```python
from build123d import *

# Parameters (mm, degrees)
SKETCH1_W                = 75
SKETCH1_H                = 40
SKETCH1_R                = 5
SKETCH1_R_2              = 1.7
SKETCH1_R_3              = 1.197563381
SKETCH1_W_2              = 5
SKETCH1_H_2              = 20
BOSS_EXTRUDE1_DEPTH      = 3
CUT_EXTRUDE1_DEPTH       = 43.605750786
CUT_EXTRUDE1_DEPTH_BACK  = 43.605750786
SKETCH2_W                = 67
SKETCH2_H                = 28
BOSS_EXTRUDE3_DEPTH      = 75
BOSS_EXTRUDE3_DEPTH_BACK = 3
SKETCH6_W                = 67
SKETCH6_H                = 11
CUT_EXTRUDE4_DEPTH       = 91.863909227
SKETCH7_W                = 70
SKETCH7_H                = 37
BOSS_EXTRUDE4_DEPTH      = 6
SKETCH8_W                = 6
SKETCH8_H                = 62
CUT_EXTRUDE6_DEPTH       = 29
SKETCH9_R                = 1.25
SKETCH9_R_2              = 10.5
CUT_EXTRUDE8_DEPTH       = 122.975407357
SKETCH11_W               = 6
SKETCH11_H               = 4
CUT_EXTRUDE9_DEPTH       = 114.473565204
SKETCH12_W               = 35
SKETCH12_H               = 4
BOSS_EXTRUDE5_DEPTH      = 70
SKETCH13_R               = 5
SKETCH13_R_2             = 1.7
CUT_EXTRUDE11_DEPTH      = 10


with BuildPart() as part:
    # Sketch1 → Boss-Extrude1 (new body)
    with BuildSketch(Plane(origin=(0, 0, 0), x_dir=(1, 0, 0), z_dir=(0, 1, 0))):
        Rectangle(SKETCH1_W, SKETCH1_H)
        with Locations(Location((-21, 0, 0), (0, 0, 270))):
            Circle(SKETCH1_R, mode=Mode.SUBTRACT)
        with Locations(Location((-30, 8.25, 0), (0, 0, 270))):
            Circle(SKETCH1_R_2, mode=Mode.SUBTRACT)
        with Locations(Location((-12, 8.25, 0), (0, 0, 270))):
            Circle(SKETCH1_R_2, mode=Mode.SUBTRACT)
        with Locations(Location((-12, -8.25, 0), (0, 0, 270))):
            Circle(SKETCH1_R_2, mode=Mode.SUBTRACT)
        with Locations(Location((-30, -8.25, 0), (0, 0, 270))):
            Circle(SKETCH1_R_2, mode=Mode.SUBTRACT)
        with Locations(Location((12, 8.25, 0), (0, 0, 90))):
            Circle(SKETCH1_R_2, mode=Mode.SUBTRACT)
        with Locations(Location((12, -8.25, 0), (0, 0, 90))):
            Circle(SKETCH1_R_2, mode=Mode.SUBTRACT)
        with Locations(Location((21, 0, 0), (0, 0, 90))):
            Circle(SKETCH1_R, mode=Mode.SUBTRACT)
        with Locations(Location((30, -8.25, 0), (0, 0, 90))):
            Circle(SKETCH1_R_2, mode=Mode.SUBTRACT)
        with Locations(Location((30, 8.25, 0), (0, 0, 90))):
            Circle(SKETCH1_R_2, mode=Mode.SUBTRACT)
        with Locations(Location((-30, -17.5, 0), (0, 0, 270))):
            Circle(SKETCH1_R_3, mode=Mode.SUBTRACT)
        with Locations(Location((-13.5, -17.5, 0), (0, 0, 270))):
            Circle(SKETCH1_R_3, mode=Mode.SUBTRACT)
        with Locations(Location((13.5, -17.5, 0), (0, 0, 90))):
            Circle(SKETCH1_R_3, mode=Mode.SUBTRACT)
        with Locations(Location((30, -17.5, 0), (0, 0, 90))):
            Circle(SKETCH1_R_3, mode=Mode.SUBTRACT)
        with Locations(Location((30, 17.5, 0), (0, 0, 270))):
            Circle(SKETCH1_R_3, mode=Mode.SUBTRACT)
        with Locations(Location((13.5, 17.5, 0), (0, 0, 270))):
            Circle(SKETCH1_R_3, mode=Mode.SUBTRACT)
        with Locations(Location((-13.5, 17.5, 0), (0, 0, 90))):
            Circle(SKETCH1_R_3, mode=Mode.SUBTRACT)
        with Locations(Location((-30, 17.5, 0), (0, 0, 90))):
            Circle(SKETCH1_R_3, mode=Mode.SUBTRACT)
        Rectangle(SKETCH1_W_2, SKETCH1_H_2, mode=Mode.SUBTRACT)
    extrude(amount=BOSS_EXTRUDE1_DEPTH)

    # Sketch2 → Cut-Extrude1 (cut, two sides: drawn at the far end of the back side and taken through both)
    with BuildSketch(Plane(origin=(0, 3, 0), x_dir=(1, 0, 0), z_dir=(0, 1, 0)).offset(-CUT_EXTRUDE1_DEPTH_BACK)):
        Rectangle(SKETCH2_W, SKETCH2_H)
    extrude(amount=CUT_EXTRUDE1_DEPTH + CUT_EXTRUDE1_DEPTH_BACK, mode=Mode.SUBTRACT)

    # Sketch3 → Boss-Extrude3 (add, two sides: drawn at the far end of the back side and taken through both)
    with BuildSketch(Plane(origin=(0, 3, 0), x_dir=(1, 0, 0), z_dir=(0, 1, 0)).offset(-BOSS_EXTRUDE3_DEPTH_BACK)):
        Polygon((37.5, -35), (37.5, -20), (33.5, -20), (-33.5, -20), (-37.5, -20), (-37.5, -35), align=None)
        Polygon((33.5, 20), (37.5, 20), (37.5, 35), (-37.5, 35), (-37.5, 20), (-33.5, 20), align=None)
        Polygon((37.5, -20), (37.5, 20), (33.5, 20), (33.5, 14), (33.5, -14), (33.5, -20), align=None)
        Polygon((-33.5, 14), (-33.5, 20), (-37.5, 20), (-37.5, -20), (-33.5, -20), (-33.5, -14), align=None)
    extrude(amount=BOSS_EXTRUDE3_DEPTH + BOSS_EXTRUDE3_DEPTH_BACK)

    # Sketch6 → Cut-Extrude4 (cut, through all)
    with BuildSketch(Plane(origin=(0, 3, 0), x_dir=(1, 0, 0), z_dir=(0, 1, 0))):
        with Locations((0, -25.5)):
            Rectangle(SKETCH6_W, SKETCH6_H)
        with Locations((0, 25.5)):
            Rectangle(SKETCH6_W, SKETCH6_H)
    extrude(amount=CUT_EXTRUDE4_DEPTH, mode=Mode.SUBTRACT)

    # Sketch7 → Boss-Extrude4 (add)
    with BuildSketch(Plane.ZY.offset(37.5)):
        with Locations((0, 59.5)):
            Rectangle(SKETCH7_W, SKETCH7_H)
    boss_extrude4 = extrude(amount=BOSS_EXTRUDE4_DEPTH)

    # Mirror2: Boss-Extrude4 across plane
    add(boss_extrude4.mirror(Plane(origin=(0, 0, 0), x_dir=(0, 0, 1), z_dir=(1, 0, 0))))

    # Sketch8 → Cut-Extrude6 (cut)
    with BuildSketch(Plane(origin=(0, 78, 0), x_dir=(1, 0, 0), z_dir=(0, 1, 0))):
        with Locations((-36.5, 0)):
            Rectangle(SKETCH8_W, SKETCH8_H)
        with Locations((36.5, 0)):
            Rectangle(SKETCH8_W, SKETCH8_H)
    extrude(amount=-CUT_EXTRUDE6_DEPTH, mode=Mode.SUBTRACT)

    # Sketch9 → Cut-Extrude8 (cut, through all)
    with BuildSketch(Plane.ZY.offset(43.5)):
        with Locations((-27.75, 74.75)):
            Circle(SKETCH9_R)
        with Locations((-27.75, 52.75)):
            Circle(SKETCH9_R)
        with Locations((4.25, 63.75)):
            Circle(SKETCH9_R_2)
        with Locations((12.25, 52.75)):
            Circle(SKETCH9_R)
        with Locations((12.25, 74.75)):
            Circle(SKETCH9_R)
    extrude(amount=-CUT_EXTRUDE8_DEPTH, mode=Mode.SUBTRACT)

    # Sketch11 → Cut-Extrude9 (cut, through all)
    with BuildSketch(Plane.XY.offset(35)):
        with Locations((-40.5, 43)):
            Rectangle(SKETCH11_W, SKETCH11_H)
        with Locations((40.5, 43)):
            Rectangle(SKETCH11_W, SKETCH11_H)
    extrude(amount=-CUT_EXTRUDE9_DEPTH, mode=Mode.SUBTRACT)

    # Sketch12 → Boss-Extrude5 (add)
    with BuildSketch(Plane.XY.offset(35)):
        with Locations((-55, 20.5)):
            Rectangle(SKETCH12_W, SKETCH12_H)
    boss_extrude5 = extrude(amount=-BOSS_EXTRUDE5_DEPTH)

    # Mirror3: Boss-Extrude5 across plane
    add(boss_extrude5.mirror(Plane(origin=(0, 0, 0), x_dir=(0, 0, 1), z_dir=(1, 0, 0))))

    # Sketch13 → Cut-Extrude11 (cut)
    with BuildSketch(Plane(origin=(0, 22.5, 0), x_dir=(1, 0, 0), z_dir=(0, 1, 0))):
        with Locations(Location((-60, 0, 0), (0, 0, 270))):
            Circle(SKETCH13_R)
        with Locations(Location((-68.25, 9, 0), (0, 0, 270))):
            Circle(SKETCH13_R_2)
        with Locations(Location((-51.75, 9, 0), (0, 0, 270))):
            Circle(SKETCH13_R_2)
        with Locations(Location((-51.75, -9, 0), (0, 0, 270))):
            Circle(SKETCH13_R_2)
        with Locations(Location((-68.25, -9, 0), (0, 0, 270))):
            Circle(SKETCH13_R_2)
        with Locations((68.25, -9)):
            Circle(SKETCH13_R_2)
        with Locations((51.75, -9)):
            Circle(SKETCH13_R_2)
        with Locations((51.75, 9)):
            Circle(SKETCH13_R_2)
        with Locations((68.25, 9)):
            Circle(SKETCH13_R_2)
        with Locations((60, 0)):
            Circle(SKETCH13_R)
    extrude(amount=-CUT_EXTRUDE11_DEPTH, mode=Mode.SUBTRACT)


solid = part.part
```
Geometry: final body of the model. Coordinates: model frame, mm. A direction names the side the tool comes from. Coordinates: 2 decimals unless noted, no trailing zeros. Order: outer loops, then holes, each group sorted by start corner. A loop starts at its lowest first (then second) coordinate and runs counter-clockwise, first axis right, second up. Notation, with made-up numbers: M 34,-38 L 51,-38 A26 cw 51,-19 Z; hole C -13,-14.75 d7. An arc over 180 degrees is marked long. Answer as CSV lines item,"result".
Q1. Draft query along Y for faces 1 (the flat face through (-1, 38, -35)), 2 (the flat face through (37.5, 34, 0)), 3 (the flat face through (-51, 18.5, 0)). Return one class per face: pulls with the +Y half, pulls with the -Y half, needs draft (parallel to the pull), parting line crosses it, or undercut.
Answers:
face 1,"needs draft"
face 2,"undercut"
face 3,"pulls with the -Y half"
Q2. Section B-B on x = 68.25. Return the cut outline in (y, z).
Answers:
outline,"M 18.5,-35 L 22.5,-35 L 22.5,-10.7 L 18.5,-10.7 Z; M 18.5,-7.3 L 22.5,-7.3 L 22.5,7.3 L 18.5,7.3 Z; M 18.5,10.7 L 22.5,10.7 L 22.5,35 L 18.5,35 Z"
Q3. Section A-A on y = 27.5. Return the cut outline in (x, z), and give its area (3 significant figures).
Answers:
outline,"M -37.5,-35 L 37.5,-35 L 37.5,35 L -37.5,35 Z; hole M -33.5,-31 L 33.5,-31 L 33.5,31 L -33.5,31 Z"
area,"1,100 mm^2"
Q4. Section D-D on z = 9. Count the separate pieces of the cut face and the enclosed holes in it, and give its area (3 significant figures).
Answers:
separate pieces,"8"
enclosed holes,"0"
area,"748 mm^2"
Q5. Set-up query: faces 4 (the flat face through (40, 45, 0)), 5 (the flat face through (39.5, 63.7, -6.5)), 6 (the flat face through (-41, 45, 0)), 7 (the flat face through (43.5, 62, -8)). Return all of +Z, -Z, +X, -X, +Y, -Y with unobstructed straight access to the full face (end or side cutting, diameter ignored); none if empty.
Answers:
face 4,"+Z, -Z, +X"
face 5,"+Y"
face 6,"+Z, -Z, -X"
face 7,"+Z, -Z, +X, +Y"
Q6. Line query: probe 1 along X at (y, z) = (2.25, 17.5); probe 2 along X at (y, z) = (20.4, 9); probe 3 along X at (y, z) = (21.2, 0). Output: solid intervals per line, ascending. Write a range as [from, to].
Answers:
probe 1,"x = [-37.5, -31.2], [-28.8, -14.7], [-12.3, 12.3], [14.7, 28.8], [31.2, 37.5]"
probe 2,"x = [-72.5, -69.95], [-66.55, -53.45], [-50.05, -33.5], [33.5, 50.05], [53.45, 66.55], [69.95, 72.5]"
probe 3,"x = [-72.5, -65], [-55, -33.5], [33.5, 55], [65, 72.5]"
Q7. Section C-C on x = -4. Return the cut outline in (y, z).
Answers:
outline,"M 0,-35 L 78,-35 L 78,-31 L 3,-31 L 3,-14 L 0,-14 Z; M 0,14 L 3,14 L 3,31 L 78,31 L 78,35 L 0,35 Z"
Q8. First-contact query: P1, Ø12, axis at y = 44.5, z = -8.5, coming from the +X side; P2, Ø5, axis at x = -46.5, z = 24.5, coming from the +Y side; P3, Ø2, axis at y = 11.5, z = -17, coming from the -X side; P4, Ø1.9, axis at x = 30, z = -17.5, coming from the -Y side. Flat tips, straight axial feed; report the tip coordinate or a pass-through.
Answers:
P1,"stops at x = 43.5"
P2,"stops at y = 22.5"
P3,"stops at x = -37.5"
P4,"passes through"
